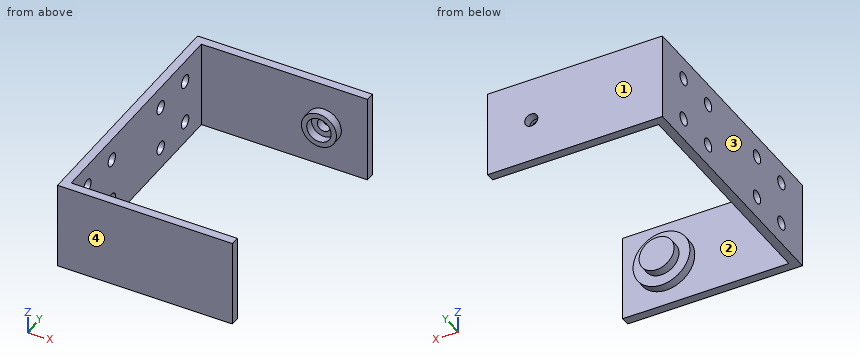
from build123d import *

# Parameters (mm, degrees)
SKETCH1_R                 = 6.5
SKETCH1_R_2               = 4
SKETCH1_R_3               = 2.8
SKETCH1_R_4               = 1.5
BOSS_EXTRUDE1_DEPTH       = 2
BOSS_EXTRUDE2_START       = 2
SKETCH1_3_R               = 4
SKETCH1_3_R_2             = 2.8
SKETCH1_3_R_3             = 1.5
BOSS_EXTRUDE2_DEPTH       = 2
SKETCH1_4_W               = 40
SKETCH1_4_H               = 20
BOSS_EXTRUDE3_DEPTH       = 2
SKETCH2_W                 = 2
SKETCH2_H                 = 20
BOSS_EXTRUDE4_DEPTH       = 53.28
BOSS_EXTRUDE5_START       = 53.28
SKETCH1_5_W               = 40
SKETCH1_5_H               = 20
SKETCH1_5_R               = 6.5
SKETCH1_5_R_2             = 4
SKETCH1_5_R_3             = 2.8
SKETCH1_5_R_4             = 1.5
BOSS_EXTRUDE5_DEPTH       = 2
BOSS_EXTRUDE6_START       = 51.28
SKETCH1_6_R               = 4
SKETCH1_6_R_2             = 2.8
BOSS_EXTRUDE6_DEPTH       = 2
F_3_0MM_DOWEL_HOLE1_D     = 3
F_3_0MM_DOWEL_HOLE1_DEPTH = 7
F_3_0MM_DOWEL_HOLE1_TIP   = 0.901290929


with BuildPart() as part:
    # Sketch1 → Boss-Extrude1 (new body)
    # profile 1 of 4: a face of its own
    with BuildSketch(Plane(origin=(0, 0, 0), x_dir=(1, 0, 0), z_dir=(0, 1, 0))):
        with Locations(Location((0, 0, 0), (0, 0, 270))):
            Circle(SKETCH1_R)
        Circle(SKETCH1_R_2, mode=Mode.SUBTRACT)
    # profile 2 of 4: a face of its own
    with BuildSketch(Plane(origin=(0, 0, 0), x_dir=(1, 0, 0), z_dir=(0, 1, 0))):
        Circle(SKETCH1_R_2)
        Circle(SKETCH1_R_3, mode=Mode.SUBTRACT)
    # profile 3 of 4: a face of its own
    with BuildSketch(Plane(origin=(0, 0, 0), x_dir=(1, 0, 0), z_dir=(0, 1, 0))):
        Circle(SKETCH1_R_3)
        Circle(SKETCH1_R_4, mode=Mode.SUBTRACT)
    # profile 4 of 4: a face of its own
    with BuildSketch(Plane(origin=(0, 0, 0), x_dir=(1, 0, 0), z_dir=(0, 1, 0))):
        Circle(SKETCH1_R_4)
    extrude(amount=BOSS_EXTRUDE1_DEPTH)

    # Sketch1<3> → Boss-Extrude2 (add)
    # profile 1 of 3: a face of its own
    with BuildSketch(Plane(origin=(0, 0, 0), x_dir=(1, 0, 0), z_dir=(0, 1, 0)).offset(BOSS_EXTRUDE2_START)):
        with Locations(Location((0, 0, 0), (0, 0, 270))):
            Circle(SKETCH1_3_R)
        Circle(SKETCH1_3_R_2, mode=Mode.SUBTRACT)
    # profile 2 of 3: a face of its own
    with BuildSketch(Plane(origin=(0, 0, 0), x_dir=(1, 0, 0), z_dir=(0, 1, 0)).offset(BOSS_EXTRUDE2_START)):
        Circle(SKETCH1_3_R_2)
        Circle(SKETCH1_3_R_3, mode=Mode.SUBTRACT)
    # profile 3 of 3: a face of its own
    with BuildSketch(Plane(origin=(0, 0, 0), x_dir=(1, 0, 0), z_dir=(0, 1, 0)).offset(BOSS_EXTRUDE2_START)):
        Circle(SKETCH1_3_R_3)
    extrude(amount=BOSS_EXTRUDE2_DEPTH)

    # Sketch1<4> → Boss-Extrude3 (add)
    with BuildSketch(Plane(origin=(0, 0, 0), x_dir=(1, 0, 0), z_dir=(0, 1, 0))):
        with Locations((-10, 0)):
            Rectangle(SKETCH1_4_W, SKETCH1_4_H)
    extrude(amount=-BOSS_EXTRUDE3_DEPTH)

    # Sketch2 → Boss-Extrude4 (add)
    with BuildSketch(Plane(origin=(0, 0, 0), x_dir=(1, 0, 0), z_dir=(0, 1, 0))):
        with Locations((-29, 0)):
            Rectangle(SKETCH2_W, SKETCH2_H)
    extrude(amount=BOSS_EXTRUDE4_DEPTH)

    # Sketch1<5> → Boss-Extrude5 (add)
    # profile 1 of 4: a face of its own
    with BuildSketch(Plane(origin=(0, 0, 0), x_dir=(1, 0, 0), z_dir=(0, 1, 0)).offset(BOSS_EXTRUDE5_START)):
        with Locations((-10, 0)):
            Rectangle(SKETCH1_5_W, SKETCH1_5_H)
        with Locations(Location((0, 0, 0), (0, 0, 270))):
            Circle(SKETCH1_5_R, mode=Mode.SUBTRACT)
    # profile 2 of 4: a face of its own
    with BuildSketch(Plane(origin=(0, 0, 0), x_dir=(1, 0, 0), z_dir=(0, 1, 0)).offset(BOSS_EXTRUDE5_START)):
        with Locations(Location((0, 0, 0), (0, 0, 270))):
            Circle(SKETCH1_5_R)
        with Locations(Location((0, 0, 0), (0, 0, 270))):
            Circle(SKETCH1_5_R_2, mode=Mode.SUBTRACT)
    # profile 3 of 4: a face of its own
    with BuildSketch(Plane(origin=(0, 0, 0), x_dir=(1, 0, 0), z_dir=(0, 1, 0)).offset(BOSS_EXTRUDE5_START)):
        with Locations(Location((0, 0, 0), (0, 0, 270))):
            Circle(SKETCH1_5_R_2)
        Circle(SKETCH1_5_R_3, mode=Mode.SUBTRACT)
    # profile 4 of 4: a face of its own
    with BuildSketch(Plane(origin=(0, 0, 0), x_dir=(1, 0, 0), z_dir=(0, 1, 0)).offset(BOSS_EXTRUDE5_START)):
        Circle(SKETCH1_5_R_3)
        with Locations(Location((0, 0, 0), (0, 0, 270))):
            Circle(SKETCH1_5_R_4, mode=Mode.SUBTRACT)
    extrude(amount=BOSS_EXTRUDE5_DEPTH)

    # Sketch1<6> → Boss-Extrude6 (add)
    with BuildSketch(Plane(origin=(0, 0, 0), x_dir=(1, 0, 0), z_dir=(0, 1, 0)).offset(BOSS_EXTRUDE6_START)):
        with Locations(Location((0, 0, 0), (0, 0, 270))):
            Circle(SKETCH1_6_R)
        with Locations(Location((0, 0, 0), (0, 0, 90))):
            Circle(SKETCH1_6_R_2, mode=Mode.SUBTRACT)
    extrude(amount=BOSS_EXTRUDE6_DEPTH)

    # Ø3.0mm Dowel Hole1
    with Locations(Plane.ZY.offset(30)):
        with Locations((-5, 46.64), (5, 46.64), (-5, 36.64), (5, 36.64), (-5, 16.64), (5, 16.64), (-5, 6.64), (5, 6.64)):
            Hole(F_3_0MM_DOWEL_HOLE1_D / 2, depth=F_3_0MM_DOWEL_HOLE1_DEPTH)
            with Locations((0, 0, -(F_3_0MM_DOWEL_HOLE1_DEPTH + F_3_0MM_DOWEL_HOLE1_TIP / 2))):  # 118° drill point
                Cone(0, F_3_0MM_DOWEL_HOLE1_D / 2, F_3_0MM_DOWEL_HOLE1_TIP, mode=Mode.SUBTRACT)


solid = part.part
The listing builds one solid part. Answer for the finished solid, in the listing's coordinates (mm). Face numbers are marked on the shaded views. Coordinates: 2 decimals unless noted, no trailing zeros. Write each loop counter-clockwise with the first axis right and the second up, starting at its lowest first coordinate (ties: lowest second). Pieces come first, ordered by that corner, then holes. Notation, with made-up numbers: M -27,70.5 L -4,70.5 A18 ccw -4,94.5 Z; hole C 3,31.25 d3. An arc over 180 degrees is marked long. Put each result on its own line as item: value. Start each with the question number.
1. A cutting plane is placed at A-A on x = -20.5. Write down the section's boundary in (y, z).
2. Consider line 1 (Y direction, x = -29.15, z = -5); line 2 (Y direction, x = -0.5, z = -6.75); line 3 (Y direction, x = -1, z = 1.5). Determine where each line is inside the solid, lowest interval first. Write a range as from..to.
3. A flat-ended cylindrical pin translates along its axis: P1, Ø5, axis at y = 16.64, z = 5, coming from the +X side. Find the tip coordinate at first contact, or state that the pin passes through.
4. For a pull along Y with two mould halves and no side action, classify the marked faces 1, 2, 3 and 4 as pulls with the +Y half, pulls with the -Y half, needs draft (parallel to the pull), parting line crosses it, or undercut.
5. A cutting plane is placed at B-B on x = 0. Write down the section's boundary in (y, z), then the cut area to 3 significant figures.
6. A cutting plane is placed at D-D on z = -5. Write down the section's boundary in (x, y), then the cut area to 3 significant figures.
7. A cutting plane is placed at C-C on y = 46.64. Write down the section's boundary in (x, z), then the cut area to 3 significant figures.
Resolved:
1. outline: M -2,-10 L 0,-10 L 0,10 L -2,10 Z; M 53.28,-10 L 55.28,-10 L 55.28,10 L 53.28,10 Z
2. line 1: y = -2..5.14, 8.14..15.14, 18.14..35.14, 38.14..45.14, 48.14..55.28
2. line 2: y = -2..0, 53.28..55.28
2. line 3: y = -2..4, 53.28..55.28
3. P1: stops at x = -28
4. face 1: pulls with the +Y half
4. face 2: undercut
4. face 3: needs draft
4. face 4: pulls with the -Y half
5. outline: M -2,-10 L 0,-10 L 0,-6.5 L 2,-6.5 L 2,-4 L 4,-4 L 4,4 L 2,4 L 2,6.5 L 0,6.5 L 0,10 L -2,10 Z; M 51.28,-4 L 53.28,-4 L 53.28,-10 L 55.28,-10 L 55.28,-1.5 L 53.28,-1.5 L 53.28,-2.8 L 51.28,-2.8 Z; M 51.28,2.8 L 53.28,2.8 L 53.28,1.5 L 55.28,1.5 L 55.28,10 L 53.28,10 L 53.28,4 L 51.28,4 Z
5. area: 121 mm2
6. outline: M -30,-2 L 10,-2 L 10,0 L 4.15,0 L 4.15,2 L -4.15,2 L -4.15,0 L -28,0 L -28,5.14 L -30,5.14 Z; M -30,8.14 L -28,8.14 L -28,15.14 L -30,15.14 Z; M -30,18.14 L -28,18.14 L -28,35.14 L -30,35.14 Z; M -30,38.14 L -28,38.14 L -28,45.14 L -30,45.14 Z; M -30,48.14 L -28,48.14 L -28,53.28 L 10,53.28 L 10,55.28 L -30,55.28 Z
6. area: 259 mm2
7. outline: M -30,-10 L -28,-10 L -28,-6.5 L -30,-6.5 Z; M -30,-3.5 L -28,-3.5 L -28,3.5 L -30,3.5 Z; M -30,6.5 L -28,6.5 L -28,10 L -30,10 Z
7. area: 28.0 mm2
